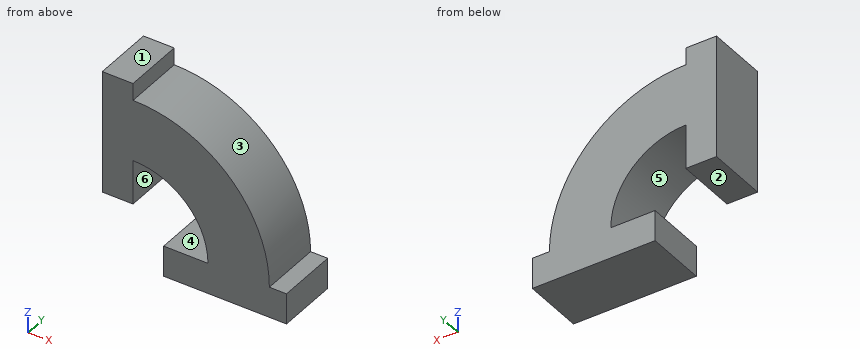
from build123d import *

# Parameters (mm, degrees)
SKETCH2_W           = 1
SKETCH2_H           = 4
SKETCH2_W_2         = 4
SKETCH2_H_2         = 1
BOSS_EXTRUDE1_DEPTH = 2


with BuildPart() as part:
    # Sketch2 → Boss-Extrude1 (new body)
    with BuildSketch(Plane(origin=(0, 0, 0), x_dir=(1, 0, 0), z_dir=(0, 1, 0))):
        with Locations((0.5, -4)):
            Rectangle(SKETCH2_W, SKETCH2_H)
        with BuildLine():
            Line((5.441670533, -1), (3.441670533, -1))
            ThreePointArc((3.441670533, -1), (2.726521791, -2.726521791), (1, -3.441670533))
            Line((1, -3.441670533), (1, -5.441670533))
            ThreePointArc((1, -5.441670533), (4.140735354, -4.140735354), (5.441670533, -1))
        make_face()
        with Locations((4, -0.5)):
            Rectangle(SKETCH2_W_2, SKETCH2_H_2)
    extrude(amount=BOSS_EXTRUDE1_DEPTH)


solid = part.part
Geometry: final body of the model. Coordinates: model frame, mm. Face numbers are marked on the shaded views. A direction names the side the tool comes from. Give positions to 0.01 mm unless a question says otherwise; leave off trailing zeros. Write each loop counter-clockwise with the first axis right and the second up, starting at its lowest first coordinate (ties: lowest second). Pieces come first, ordered by that corner, then holes. Notation, with made-up numbers: (33, 35) -> (43, 35) arc R17 ccw to (43, 46) -> close; hole circle Ø8 at (4.25, 27.5). An arc over 180 degrees is marked (long way). Answer in a Markdown table with one row per item.
(1) Pin query (flat end, axial travel): pin 1 (0.5 mm diameter, centred on y = 1, z = 0.5, fed in from -X); pin 2 (1.2 mm diameter, centred on y = 1.5, z = 2.5, fed in from +X); pin 3 (0.5 mm diameter, centred on x = 0.5, y = 0.5, fed in from -Z). Return the tip coordinate at first contact, or that it passes through.
Answers below:
| item | result |
|---|---|
| pin 1 | x = 2 |
| pin 2 | x = 5.35 |
| pin 3 | z = 2 |
(2) Section query B-B on y = 0.9. Return loops of the section in (x, z), then the cut area to 3 significant figures.
Answers below:
| item | result |
|---|---|
| outline | (0, 2) -> (1, 2) -> (1, 3.44) arc R2.44 cw to (3.44, 1) -> (2, 1) -> (2, 0) -> (6, 0) -> (6, 1) -> (5.44, 1) arc R4.44 ccw to (1, 5.44) -> (1, 6) -> (0, 6) -> close |
| area | 18.8 mm^2 |
(3) Ray query, line 1 along Z through (x, y) = (0.95, 0.7); line 2 along X through (y, z) = (0.4, 2.6). Return the intervals inside material, ascending. Write a range as [from, to].
Answers below:
| item | result |
|---|---|
| line 1 | [2, 6] |
| line 2 | [0, 1], [2.84, 5.14] |
(4) Section query C-C on x = 2.9. Return loops of the section in (y, z).
Answers below:
| item | result |
|---|---|
| outline | (0, 0) -> (2, 0) -> (2, 1) -> (0, 1) -> close; (0, 2.53) -> (2, 2.53) -> (2, 5.01) -> (0, 5.01) -> close |
(5) Section query D-D on x = 0.9. Return loops of the section in (y, z), then the cut area to 3 significant figures.
Answers below:
| item | result |
|---|---|
| outline | (0, 2) -> (2, 2) -> (2, 6) -> (0, 6) -> close |
| area | 8.00 mm^2 |
(6) Draft query along X for the marked faces 3, 4, 5 and 6. Return one class per face: +X half, -X half, draft (parallel to the pull), parting line (faces both ways), or undercut.
Answers below:
| item | result |
|---|---|
| face 3 | +X half |
| face 4 | draft |
| face 5 | undercut |
| face 6 | undercut |
(7) Set-up query: the marked faces 1 and 2. Return all of +Z, -Z, +X, -X, +Y, -Y with unobstructed straight access to the full face (end or side cutting, diameter ignored); none if empty.
Answers below:
| item | result |
|---|---|
| face 1 | +Z, +X, -X, +Y, -Y |
| face 2 | -Z, -X, +Y, -Y |
(8) Section query A-A on z = 2.75. Return loops of the section in (x, y), then the cut area to 3 significant figures.
Answers below:
| item | result |
|---|---|
| outline | (0, 0) -> (1, 0) -> (1, 2) -> (0, 2) -> close; (2.7, 0) -> (5.08, 0) -> (5.08, 2) -> (2.7, 2) -> close |
| area | 6.76 mm^2 |
